from build123d import *

# Parameters (mm, degrees)
BOSS_EXTRUDE1_DEPTH          = 7
M2_5X0_45_TAPPED_HOLE1_D     = 2.05
M2_5X0_45_TAPPED_HOLE1_DEPTH = 6.4262
M2_5X0_45_TAPPED_HOLE1_TIP   = 0.615882135
FILLET1_R                    = 1.27


with BuildPart() as part:
    # Sketch1 → Revolve1 (revolve)
    with BuildSketch(Plane(origin=(0, 0, 0), x_dir=(0, 0, -1), z_dir=(1, 0, 0))):
        Polygon((-2.5, 0), (-2.5, 5), (0, 5), (0, 14), (38, 14), (38, 0), align=None)
    revolve(axis=Axis((0, 0, 0), (0, 0, -1)))

    # Sketch2 → Boss-Extrude1 (add)
    with BuildSketch(Plane.XY.offset(2.5)):
        with BuildLine():
            Line((-1.058300524, -0.45), (1.058300524, -0.45))
            ThreePointArc((1.058300524, -0.45), (0, 1.15), (-1.058300524, -0.45))
        make_face()
    extrude(amount=BOSS_EXTRUDE1_DEPTH)

    # M2.5x0.45 Tapped Hole1
    with Locations(Plane.XY):
        with Locations((8, 0), (-8, 0)):
            Hole(M2_5X0_45_TAPPED_HOLE1_D / 2, depth=M2_5X0_45_TAPPED_HOLE1_DEPTH)
            with Locations((0, 0, -(M2_5X0_45_TAPPED_HOLE1_DEPTH + M2_5X0_45_TAPPED_HOLE1_TIP / 2))):  # 118° drill point
                Cone(0, M2_5X0_45_TAPPED_HOLE1_D / 2, M2_5X0_45_TAPPED_HOLE1_TIP, mode=Mode.SUBTRACT)

    # Fillet1
    fillet1_edges = [part.edges().sort_by_distance(p)[0] for p in [
        (0, -14, 0),
    ]]
    fillet(fillet1_edges, radius=FILLET1_R)


solid = part.part
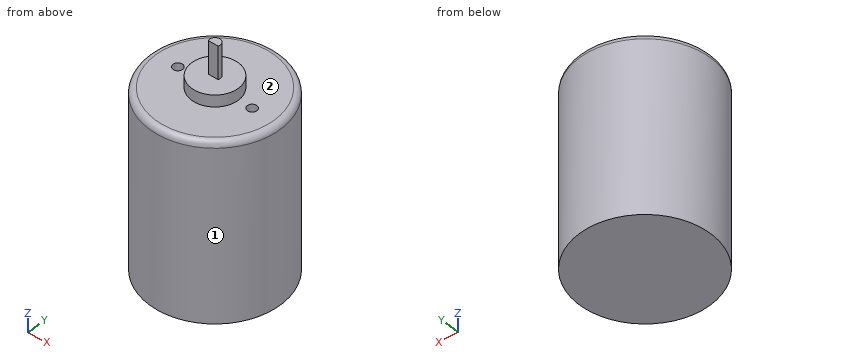
Here's how the part is built. I have some questions about the finished solid (model axes, mm). Face numbers are marked on the shaded views. A direction names the side the tool comes from. Coordinates: 2 decimals unless noted, no trailing zeros. Order: outer loops, then holes, each group sorted by start corner. A loop starts at its lowest first (then second) coordinate and runs counter-clockwise, first axis right, second up. Notation, with made-up numbers: (86.5, 27.5) - (143.5, 27.5) arc R11 cw to (143.5, 44.5) - close; hole circle Ø7 at (89, -2). An arc over 180 degrees is marked (long way). Use CSV: the item, a comma, the result in double quotes. Start each with the question number.
1. For the marked faces 1 and 2, which set-ups out of +Z, -Z, +X, -X, +Y, -Y let a thin tool reach every point of the face, with its end or its side?
2. Please list where these lines run through material, in increasing order: line 1 (X direction, y = 0, z = -1.5) (3 decimals); line 2 (Z direction, x = 9, y = 5.75); line 3 (Z direction, x = -2, y = 4.25). Write a range as from..to.
3. Suppose I cut it at C-C on z = 6. List the corners of the cut face in (x, y) for me, then the cut area to 3 significant figures.
4. I'm going to push flat-ended pins straight in: pin 1 (2 mm diameter, centred on x = -4, z = -29, fed in from -Y); pin 2 (1 mm diameter, centred on x = 11, z = -30.5, fed in from -Y); pin 3 (1.1 mm diameter, centred on x = 0, z = 6, fed in from -Y). Where does each tip first touch, or does it pass through?
5. Suppose I cut it at A-A on x = 0. List the corners of the cut face in (y, z) for me, then the cut area to 3 significant figures.
6. Suppose I cut it at B-B on z = -20. List the corners of the cut face in (x, y) for me.
Output:
1,face 1,"+Z, -Z"
1,face 2,"+Z"
2,line 1,"x = -14..-9.025, -6.975..6.975, 9.025..14"
2,line 2,"z = -38..0"
2,line 3,"z = -38..2.5"
3,outline,"(-1.06, -0.45) - (1.06, -0.45) arc R1.15 ccw (long way) to start"
3,area,"3.09 mm2"
4,pin 1,"stops at y = -13.67"
4,pin 2,"stops at y = -9.26"
4,pin 3,"stops at y = -0.45"
5,outline,"(-14, -38) - (14, -38) - (14, -1.27) arc R1.27 ccw to (12.73, 0) - (5, 0) - (5, 2.5) - (1.15, 2.5) - (1.15, 9.5) - (-0.45, 9.5) - (-0.45, 2.5) - (-5, 2.5) - (-5, 0) - (-12.73, 0) arc R1.27 ccw to (-14, -1.27) - close"
5,area,"1,100 mm2"
6,outline,"circle Ø28 at (0, 0)"
